```python
from build123d import *

# Parameters (mm, degrees)
F1_DEPTH = 35
F2_R     = 5
F3_T     = -0.6


with BuildPart() as f1:
    # F0 (on Top) → F1 (new body)
    with BuildSketch(Plane.XY):
        with BuildLine():
            Line((5.35, 6.9), (-5.35, 6.9))
            ThreePointArc((-5.35, 6.9), (-12.25, 0), (-5.35, -6.9))
            Line((-5.35, -6.9), (5.35, -6.9))
            ThreePointArc((5.35, -6.9), (12.25, 0), (5.35, 6.9))
        make_face()
    extrude(amount=F1_DEPTH)

    # F2
    f2_edges = [f1.edges().sort_by_distance(p)[0] for p in [
        (0, -6.9, 35),
    ]]
    fillet(f2_edges, radius=F2_R)

    # F3
    f3_openings = [f1.faces().sort_by_distance(p)[0] for p in [
        (0, 0, 0),
    ]]
    offset(amount=F3_T, openings=f3_openings)


solid = f1.part
```
Here's how the part is built. I have some questions about the finished solid (model axes, mm). A direction names the side the tool comes from. Give positions to 0.01 mm unless a question says otherwise; leave off trailing zeros. Write each loop counter-clockwise with the first axis right and the second up, starting at its lowest first coordinate (ties: lowest second). Pieces come first, ordered by that corner, then holes. Notation, with made-up numbers: M 7.25,-4.5 L 21.25,-4.5 A29 ccw 21.25,27.5 Z; hole C 32,73.25 d10. An arc over 180 degrees is marked long. Put each result on its own line as item: value. Start each with the question number.
Item 1: On a 3-axis mill with a long thin cutter (end or side, diameter ignored), from which of +Z, -Z, +X, -X, +Y, -Y can I reach the whole of each face in a straight line? I mean faces 1 (the flat face through (0, -6.9, 15)), 2 (the flat face through (0, -6.3, 15)). Say none if no direction works.
Item 2: I need wall thicknesses on L1, parallel to Y at x = -2.5, z = 20; L2, parallel to X at y = -0.25, z = 12.5; L3, parallel to X at y = 5, z = 11.5 (3 decimals). Which ranges of each line are inside material? Lowest first, please. Write a range as from..to.
Item 3: Thinking about a two-plate mould opening in Y: for faces 3 (the flat face through (0, 0, 34.4)), 4 (the cylindrical face through (-12.25, 0.15, 14.79)), 5 (the cylindrical face through (0.07, -5.47, 33.5)), 6 (the cylindrical face through (11.65, -0.14, 14.79)), which applies, +Y half, -Y half, draft (parallel to the pull), parting line (faces both ways), or undercut?
Item 4: If we section it at A-A, the plane z = 25.5: Write out the boundary of the cut face in (x, y), then the cut area to 3 significant figures.
Item 5: Will these pins go through, and if not, where does the flat tip stop? pin 1 (3 mm diameter, centred on y = -0.5, z = 20.5, fed in from +X); pin 2 (1.5 mm diameter, centred on x = 5, y = 4.5, fed in from +Z); pin 3 (3 mm diameter, centred on x = -2, y = 0, fed in from -Z); pin 4 (3 mm diameter, centred on y = 4.5, z = 6.5, fed in from +X).
Item 6: If we section it at B-B, the plane x = 4.5: Write out the boundary of the cut face in (y, z), then the cut area to 3 significant figures.
Values:
1. face 1: +Z, -Z, +X, -X, -Y
1. face 2: -Z
2. L1: -6.9..-6.3, 6.3..6.9
2. L2: -12.25..-11.65, 11.65..12.25
2. L3: -10.105..-9.183, 9.183..10.105
3. face 3: undercut
3. face 4: parting line
3. face 5: -Y half
3. face 6: undercut
4. outline: M -5.35,-6.9 L 5.35,-6.9 A6.9 ccw 5.35,6.9 L -5.35,6.9 A6.9 ccw Z; hole M -5.35,-6.3 L 5.35,-6.3 A6.3 ccw 5.35,6.3 L -5.35,6.3 A6.3 ccw Z
4. area: 37.7 mm²
5. pin 1: x = 12.25
5. pin 2: z = 34.65
5. pin 3: z = 34.4
5. pin 4: x = 11.56
6. outline: M -6.9,0 L -6.3,0 L -6.3,30 A4.4 cw -1.9,34.4 L 1.9,34.4 A4.4 cw 6.3,30 L 6.3,0 L 6.9,0 L 6.9,30 A5 ccw 1.9,35 L -1.9,35 A5 ccw -6.9,30 Z
6. area: 47.1 mm²
